from build123d import *

# Parameters (mm, degrees)
CUT_EXTRUDE1_REACH             = 58.627
SKETCH2_R                      = 12.5
CUT_EXTRUDE1_DIRECTION_2_REACH = 58.627
CUT_EXTRUDE2_REACH             = 41.149
CUT_EXTRUDE2_END_RADIUS        = 12.5
SKETCH3_R                      = 5.5
CHAMFER1_SIZE                  = 1


with BuildPart() as part:
    # Sketch1 → Revolve1 (revolve)
    with BuildSketch(Plane.XY, mode=Mode.PRIVATE) as revolve1_sk:
        Polygon((0, 55.5), (7.95, 55.5), (7.95, 18), (4, 18), (4, 15), (4.925, 15), (4.925, 0), (0, 0), align=None)
    revolve(revolve1_sk.sketch.rotate(Axis((0, 0, 0), (0, 1, 0)), 90), axis=Axis((0, 0, 0), (0, 1, 0)))

    # Sketch2 → Cut-Extrude1 (cut, up to next)
    with BuildSketch(Plane(origin=(0, 0, 0), x_dir=(0, 0, -1), z_dir=(1, 0, 0)), mode=Mode.PRIVATE) as cut_extrude1_sk1:
        with Locations((-12.5, 38)):
            Circle(SKETCH2_R)
    cut_extrude1_tool1 = extrude(cut_extrude1_sk1.sketch, amount=-CUT_EXTRUDE1_REACH, mode=Mode.PRIVATE) & part.part
    add(cut_extrude1_tool1.solids().sort_by_distance((0, 38, 12.5))[0], mode=Mode.SUBTRACT)

    # Sketch2 → Cut-Extrude1 direction 2 (cut, up to next)
    with BuildSketch(Plane(origin=(0, 0, 0), x_dir=(0, 0, -1), z_dir=(1, 0, 0)), mode=Mode.PRIVATE) as cut_extrude1_direction_2_sk1:
        with Locations((-12.5, 38)):
            Circle(SKETCH2_R)
    cut_extrude1_direction_2_tool1 = extrude(cut_extrude1_direction_2_sk1.sketch, amount=CUT_EXTRUDE1_DIRECTION_2_REACH, mode=Mode.PRIVATE) & part.part
    add(cut_extrude1_direction_2_tool1.solids().sort_by_distance((0, 38, 12.5))[0], mode=Mode.SUBTRACT)

    # Cut-Extrude2: up to this cylinder (the profile starts outside it)
    cut_extrude2_end = Plane(origin=(0, 38, 12.5), z_dir=(-1, 0, 0)) * Cylinder(CUT_EXTRUDE2_END_RADIUS, 108.298, mode=Mode.PRIVATE)
    # Sketch3 → Cut-Extrude2 (cut, up to the surface)
    with BuildSketch(Plane.XZ.offset(-18), mode=Mode.PRIVATE) as cut_extrude2_sk1:
        with Locations((0, 11.5)):
            Circle(SKETCH3_R)
    cut_extrude2_tool1 = extrude(cut_extrude2_sk1.sketch, amount=-CUT_EXTRUDE2_REACH, mode=Mode.PRIVATE) - cut_extrude2_end
    add(cut_extrude2_tool1.solids().sort_by_distance((0, 18, 11.5))[0], mode=Mode.SUBTRACT)

    # Chamfer1
    chamfer1_edges = [part.edges().sort_by_distance(p)[0] for p in [
        (0, 55.5, 7.95),
    ]]
    chamfer(chamfer1_edges, length=CHAMFER1_SIZE)


solid = part.part
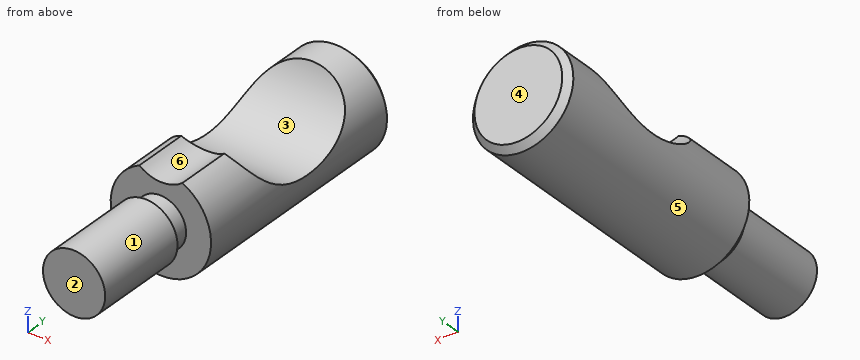
Can you work these out from the model? Positions are in its coordinate system, mm. Face numbers are marked on the shaded views. A direction names the side the tool comes from. Coordinates: 2 decimals unless noted, no trailing zeros. Write each loop counter-clockwise with the first axis right and the second up, starting at its lowest first coordinate (ties: lowest second). Pieces come first, ordered by that corner, then holes. Notation, with made-up numbers: (-17.75, 31.5) - (-7.75, 31.5) arc R9 cw to (-7.75, 36.5) - close; hole circle Ø6 at (62, 20.5). An arc over 180 degrees is marked (long way). Return JSON: item names as keys, results as strings. Group by question number.
Item 1: We'd pull the mould along Y, two halves only. Please class the marked faces 1, 2, 3 and 4: pulls with the +Y half, pulls with the -Y half, needs draft (parallel to the pull), parting line crosses it, or undercut.
Item 2: Please list where these lines run through material, in increasing order: probe 1 along Y at (x, z) = (-4.5, -1); probe 2 along Y at (x, z) = (2, -5.75); probe 3 along Y at (x, z) = (-5.5, 4.5).
Item 3: If we section it at A-A (x = 0): Write out the boundary of the cut face in (y, z) (3 decimals), then the cut area to 3 significant figures.
Item 4: Which directions (+Z, -Z, +X, -X, +Y, -Y) give clear straight access to the entire face, cutting with the end or side of a thin tool? Please do the marked faces 5 and 6.
Item 5: If we section it at B-B (y = 4): Write out the boundary of the cut face in (x, z) (3 decimals).
Item 6: I'm going to push flat-ended pins straight in: pin 1 Ø8 at (x, y) = (4.5, 7) entering from -Z; pin 2 Ø6 at (x, y) = (0.5, 44.5) entering from +Z; pin 3 Ø6 at (x, y) = (6.5, 38) entering from -Z. Where does each tip first touch, or does it pass through?
Return value:
{
 "1": {"face 1": "needs draft", "face 2": "pulls with the -Y half", "face 3": "undercut", "face 4": "pulls with the +Y half"},
 "2": {"probe 1": "y = 0 to 15, 18 to 55.5", "probe 2": "y = 18 to 55.5", "probe 3": "y = 18 to 28.4, 47.6 to 55.34"},
 "3": {"outline": "(0, -4.925) - (15, -4.925) - (15, -4) - (18, -4) - (18, -7.95) - (54.5, -7.95) - (55.5, -6.95) - (55.5, 6.95) - (54.5, 7.95) - (49.642, 7.95) arc R12.5 cw to (27.323, 6) - (18, 6) - (18, 4) - (15, 4) - (15, 4.925) - (0, 4.925) - close", "area": "616 mm^2"},
 "4": {"face 5": "+Y, -Y", "face 6": "+Z, -Y"},
 "5": {"outline": "circle Ø9.85 at (0, 0)"},
 "6": {"pin 1": "stops at z = -4.9", "pin 2": "stops at z = 4.38", "pin 3": "stops at z = -7.14"}
}
